Read the model definition and answer for the solid it produces. Units are mm, in the model's axes. Coordinates: 2 decimals unless noted, no trailing zeros. Write each loop counter-clockwise with the first axis right and the second up, starting at its lowest first coordinate (ties: lowest second). Pieces come first, ordered by that corner, then holes.
(1) Find the intervals of material crossed by probe 1 along Z at (x, y) = (1.27, 1.15) (3 decimals); probe 2 along Z at (x, y) = (3.5, 0.4), in increasing order.
(2) Section D-D on x = -3.75 is taken. Write down the section's boundary in (y, z), then the cut area to 3 significant figures.
(3) Section C-C on y = 1.25 is taken. State how many separate pieces and enclosed holes the cut face has, then the cut area to 3 significant figures.
(4) Section A-A on z = -3.81 is taken. Write down the section's boundary in (x, y) (3 decimals).
(5) The mould has two halves that part along Z. Classify faces 1 (the flat face through (0, 0, 0)), 2 (the flat face through (0, 1, 4.81)), 3 (the cylindrical face through (3.67, 0.74, 4.43)), 4 (the flat face through (0, 1, -4.81)): +Z half, -Z half, draft (parallel to the pull), parting line (faces both ways), or undercut.
(6) Section B-B on x = 3.81 is taken. Write down the section's boundary in (y, z) (3 decimals).
from build123d import *

# Parameters (mm, degrees)
SKETCH1_W           = 14.7
SKETCH1_H           = 9.62
SKETCH1_R           = 0.635
BOSS_EXTRUDE2_DEPTH = 1.5


with BuildPart() as part:
    # Sketch1 → Boss-Extrude2 (new body)
    with BuildSketch(Plane(origin=(0, 0, 0), x_dir=(1, 0, 0), z_dir=(0, 1, 0))):
        Rectangle(SKETCH1_W, SKETCH1_H)
        with Locations((-6.35, 3.81)):
            Circle(SKETCH1_R, mode=Mode.SUBTRACT)
        with Locations((-3.81, 3.81)):
            Circle(SKETCH1_R, mode=Mode.SUBTRACT)
        with Locations((-1.27, 3.81)):
            Circle(SKETCH1_R, mode=Mode.SUBTRACT)
        with Locations((1.27, 3.81)):
            Circle(SKETCH1_R, mode=Mode.SUBTRACT)
        with Locations((3.81, 3.81)):
            Circle(SKETCH1_R, mode=Mode.SUBTRACT)
        with Locations((6.35, 3.81)):
            Circle(SKETCH1_R, mode=Mode.SUBTRACT)
        with Locations((-6.35, 1.27)):
            Circle(SKETCH1_R, mode=Mode.SUBTRACT)
        with Locations((-3.81, 1.27)):
            Circle(SKETCH1_R, mode=Mode.SUBTRACT)
        with Locations((-1.27, 1.27)):
            Circle(SKETCH1_R, mode=Mode.SUBTRACT)
        with Locations((1.27, 1.27)):
            Circle(SKETCH1_R, mode=Mode.SUBTRACT)
        with Locations((3.81, 1.27)):
            Circle(SKETCH1_R, mode=Mode.SUBTRACT)
        with Locations((6.35, 1.27)):
            Circle(SKETCH1_R, mode=Mode.SUBTRACT)
        with Locations((-6.35, -1.27)):
            Circle(SKETCH1_R, mode=Mode.SUBTRACT)
        with Locations((-3.81, -1.27)):
            Circle(SKETCH1_R, mode=Mode.SUBTRACT)
        with Locations((-1.27, -1.27)):
            Circle(SKETCH1_R, mode=Mode.SUBTRACT)
        with Locations((1.27, -1.27)):
            Circle(SKETCH1_R, mode=Mode.SUBTRACT)
        with Locations((3.81, -1.27)):
            Circle(SKETCH1_R, mode=Mode.SUBTRACT)
        with Locations((6.35, -1.27)):
            Circle(SKETCH1_R, mode=Mode.SUBTRACT)
        with Locations((-6.35, -3.81)):
            Circle(SKETCH1_R, mode=Mode.SUBTRACT)
        with Locations((-3.81, -3.81)):
            Circle(SKETCH1_R, mode=Mode.SUBTRACT)
        with Locations((-1.27, -3.81)):
            Circle(SKETCH1_R, mode=Mode.SUBTRACT)
        with Locations((1.27, -3.81)):
            Circle(SKETCH1_R, mode=Mode.SUBTRACT)
        with Locations((3.81, -3.81)):
            Circle(SKETCH1_R, mode=Mode.SUBTRACT)
        with Locations((6.35, -3.81)):
            Circle(SKETCH1_R, mode=Mode.SUBTRACT)
    extrude(amount=BOSS_EXTRUDE2_DEPTH)


solid = part.part
Response:
1. probe 1: z = -4.81 to -4.445, -3.175 to -1.905, -0.635 to 0.635, 1.905 to 3.175, 4.445 to 4.81
1. probe 2: z = -4.81 to -4.36, -3.26 to -1.82, -0.72 to 0.72, 1.82 to 3.26, 4.36 to 4.81
2. outline: (0, -4.81) - (1.5, -4.81) - (1.5, -4.44) - (0, -4.44) - close; (0, -3.18) - (1.5, -3.18) - (1.5, -1.9) - (0, -1.9) - close; (0, -0.64) - (1.5, -0.64) - (1.5, 0.64) - (0, 0.64) - close; (0, 1.9) - (1.5, 1.9) - (1.5, 3.18) - (0, 3.18) - close; (0, 4.44) - (1.5, 4.44) - (1.5, 4.81) - (0, 4.81) - close
2. area: 6.84 mm2
3. separate pieces: 1
3. enclosed holes: 24
3. area: 111 mm2
4. outline: (-7.35, 0) - (-6.985, 0) - (-6.985, 1.5) - (-7.35, 1.5) - close; (-5.715, 0) - (-4.445, 0) - (-4.445, 1.5) - (-5.715, 1.5) - close; (-3.175, 0) - (-1.905, 0) - (-1.905, 1.5) - (-3.175, 1.5) - close; (-0.635, 0) - (0.635, 0) - (0.635, 1.5) - (-0.635, 1.5) - close; (1.905, 0) - (3.175, 0) - (3.175, 1.5) - (1.905, 1.5) - close; (4.445, 0) - (5.715, 0) - (5.715, 1.5) - (4.445, 1.5) - close; (6.985, 0) - (7.35, 0) - (7.35, 1.5) - (6.985, 1.5) - close
5. face 1: draft
5. face 2: +Z half
5. face 3: undercut
5. face 4: -Z half
6. outline: (0, -4.81) - (1.5, -4.81) - (1.5, -4.445) - (0, -4.445) - close; (0, -3.175) - (1.5, -3.175) - (1.5, -1.905) - (0, -1.905) - close; (0, -0.635) - (1.5, -0.635) - (1.5, 0.635) - (0, 0.635) - close; (0, 1.905) - (1.5, 1.905) - (1.5, 3.175) - (0, 3.175) - close; (0, 4.445) - (1.5, 4.445) - (1.5, 4.81) - (0, 4.81) - close
